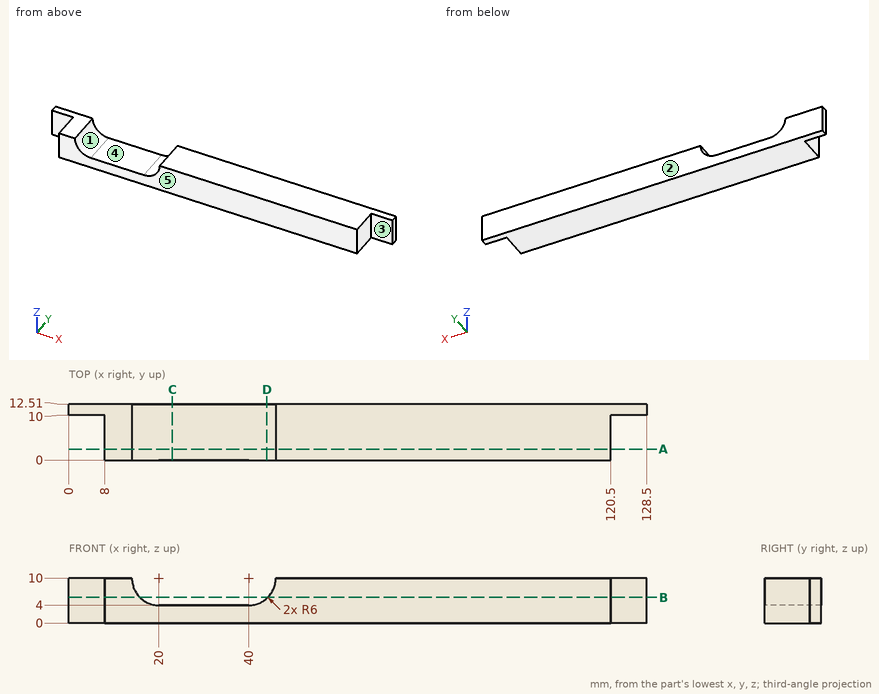
Can you work these out from the drawing? Everything is in mm from the part's minimum corner. A direction names the side the tool comes from. Give positions to 0.01 mm unless a question says otherwise; leave off trailing zeros. Loops run counter-clockwise (first coordinate to the right, second up) from the corner with the lowest first, then second, coordinate; pieces in that order, holes last. Notation, with made-up numbers: M 47.5,25 L 90.5,25 A22 cw 90.5,50 Z; hole C 65.5,-21 d4. An arc over 180 degrees is marked long. Put each result on its own line as item: value. Start each with the question number.
(1) I want a section at A-A on y = 2.5. Please give me the cut outline in (x, z), then the cut area to 3 significant figures.
(2) Will these pins go through, and if not, where does the flat tip stop? pin 1 Ø4 at (y, z) = (5.5, 3.5) entering from +X; pin 2 Ø4 at (x, z) = (124, 4) entering from -Y; pin 3 Ø6 at (y, z) = (5.5, 9) entering from -X.
(3) If we mould it in two halves opening along X, with no side actions, what happens to the marked faces 4 and 5? For each: +X half, -X half, draft (parallel to the pull), parting line (faces both ways), or undercut.
(4) I need wall thicknesses on line 1 along Y through (x, z) = (123, 3); line 2 along X through (y, z) = (2.25, 7.25); line 3 along X through (y, z) = (5, 3.5). Which ranges of each line are inside material? Lowest first, please. Write a range as [from, to].
(5) I want a section at D-D on x = 44. Please give me the cut outline in (y, z), then the cut area to 3 significant figures.
(6) I want a section at B-B on z = 5.75. Please give me the cut outline in (x, y), then the cut area to 3 significant figures.
(7) I want a section at C-C on x = 23. Please give me the cut outline in (y, z), then the cut area to 3 significant figures.
(8) For the marked faces 1, 2 and 3, which set-ups out of +Z, -Z, +X, -X, +Y, -Y let a thin tool reach every point of the face, with its end or its side?
Answer block:
1. outline: M 8,0 L 120.5,0 L 120.5,10 L 46,10 A6 cw 40,4 L 20,4 A6 cw 14,10 L 8,10 Z
1. area: 948 mm^2
2. pin 1: x = 120.5
2. pin 2: y = 10
2. pin 3: x = 8
3. face 4: undercut
3. face 5: draft
4. line 1: [10, 12.51]
4. line 2: [8, 14.67], [45.33, 120.5]
4. line 3: [8, 120.5]
5. outline: M 0,0 L 12.51,0 L 12.51,5.53 L 0,5.53 Z
5. area: 69.2 mm^2
6. outline: M 0,10 L 8,10 L 8,0 L 15.76,0 L 15.76,12.51 L 0,12.51 Z; M 44.24,0 L 120.5,0 L 120.5,10 L 128.5,10 L 128.5,12.51 L 44.24,12.51 Z
6. area: 1,090 mm^2
7. outline: M 0,0 L 12.51,0 L 12.51,4 L 0,4 Z
7. area: 50.0 mm^2
8. face 1: +Z, +Y, -Y
8. face 2: +Z, -Z, +X, -X, +Y
8. face 3: +Z, -Z, +X, -Y
